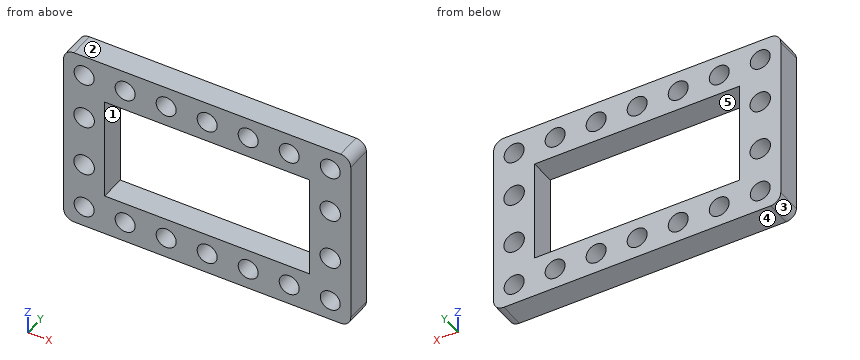
from build123d import *

# Parameters (mm, degrees)
BOSS_EXTRUDE1_DEPTH = 5
SKETCH2_R           = 1.95
SKETCH2_W           = 40
SKETCH2_H           = 20
CUT_EXTRUDE1_DEPTH  = 6
SKETCH4_W           = 22
SKETCH4_H           = 36
CUT_EXTRUDE2_DEPTH  = 10
FILLET1_R           = 2
FILLET2_R           = 2
FILLET3_R           = 2
FILLET4_R           = 2
SKETCH5_R           = 2
CUT_EXTRUDE3_DEPTH  = 6


with BuildPart() as part:
    # Sketch1 → Boss-Extrude1 (new body)
    with BuildSketch(Plane(origin=(0, 0, 0), x_dir=(1, 0, 0), z_dir=(0, 1, 0))):
        with BuildLine():
            Line((2, 0), (98, 0))
            ThreePointArc((98, 0), (99.414213562, -0.585786438), (100, -2))
            Line((100, -2), (100, -34))
            ThreePointArc((100, -34), (99.414213562, -35.414213562), (98, -36))
            Line((98, -36), (2, -36))
            ThreePointArc((2, -36), (0.585786438, -35.414213562), (0, -34))
            Line((0, -34), (0, -2))
            ThreePointArc((0, -2), (0.585786438, -0.585786438), (2, 0))
        make_face()
    extrude(amount=BOSS_EXTRUDE1_DEPTH)

    # Sketch2 → Cut-Extrude1 (cut, through all)
    with BuildSketch(Plane(origin=(0, 5, 0), x_dir=(1, 0, 0), z_dir=(0, 1, 0))):
        with Locations((90, -4.00475022)):
            Circle(SKETCH2_R)
        with Locations((82, -4.00475022)):
            Circle(SKETCH2_R)
        with Locations((18, -4.00475022)):
            Circle(SKETCH2_R)
        with Locations((26, -4.00475022)):
            Circle(SKETCH2_R)
        with Locations((34, -4.00475022)):
            Circle(SKETCH2_R)
        with Locations((42, -4.00475022)):
            Circle(SKETCH2_R)
        with Locations((50, -4.00475022)):
            Circle(SKETCH2_R)
        with Locations((58, -4.00475022)):
            Circle(SKETCH2_R)
        with Locations((66, -4.00475022)):
            Circle(SKETCH2_R)
        with Locations((74, -4.00475022)):
            Circle(SKETCH2_R)
        with Locations((90, -32)):
            Circle(SKETCH2_R)
        with Locations((82, -32)):
            Circle(SKETCH2_R)
        with Locations((18, -32)):
            Circle(SKETCH2_R)
        with Locations((26, -32)):
            Circle(SKETCH2_R)
        with Locations((34, -32)):
            Circle(SKETCH2_R)
        with Locations((42, -32)):
            Circle(SKETCH2_R)
        with Locations((50, -32)):
            Circle(SKETCH2_R)
        with Locations((58, -32)):
            Circle(SKETCH2_R)
        with Locations((66, -32)):
            Circle(SKETCH2_R)
        with Locations((74, -32)):
            Circle(SKETCH2_R)
        with Locations((50, -18)):
            Rectangle(SKETCH2_W, SKETCH2_H)
    extrude(amount=-CUT_EXTRUDE1_DEPTH, mode=Mode.SUBTRACT)

    # Sketch4 → Cut-Extrude2 (cut)
    with BuildSketch(Plane(origin=(0, 5, 0), x_dir=(1, 0, 0), z_dir=(0, 1, 0))):
        with Locations((89, -18)):
            Rectangle(SKETCH4_W, SKETCH4_H)
        with Locations((11, -18)):
            Rectangle(SKETCH4_W, SKETCH4_H)
    extrude(amount=-CUT_EXTRUDE2_DEPTH, mode=Mode.SUBTRACT)

    # Fillet1
    fillet1_edges = [part.edges().sort_by_distance(p)[0] for p in [
        (22, 2.5, 0),
    ]]
    fillet(fillet1_edges, radius=FILLET1_R)

    # Fillet2
    fillet2_edges = [part.edges().sort_by_distance(p)[0] for p in [
        (22, 2.5, 36),
    ]]
    fillet(fillet2_edges, radius=FILLET2_R)

    # Fillet3
    fillet3_edges = [part.edges().sort_by_distance(p)[0] for p in [
        (78, 2.5, 36),
    ]]
    fillet(fillet3_edges, radius=FILLET3_R)

    # Fillet4
    fillet4_edges = [part.edges().sort_by_distance(p)[0] for p in [
        (78, 2.5, 0),
    ]]
    fillet(fillet4_edges, radius=FILLET4_R)

    # Sketch5 → Cut-Extrude3 (cut, through all)
    with BuildSketch(Plane(origin=(0, 5, 0), x_dir=(1, 0, 0), z_dir=(0, 1, 0))):
        with Locations((74, -13)):
            Circle(SKETCH5_R)
        with Locations((74, -23)):
            Circle(SKETCH5_R)
        with Locations((26, -13)):
            Circle(SKETCH5_R)
        with Locations((26, -23)):
            Circle(SKETCH5_R)
    extrude(amount=-CUT_EXTRUDE3_DEPTH, mode=Mode.SUBTRACT)


solid = part.part
Can you work these out from the model? Positions are in its coordinate system, mm. Face numbers are marked on the shaded views. A direction names the side the tool comes from. Round coordinates to 2 decimals unless told otherwise and drop trailing zeros. Order: outer loops, then holes, each group sorted by start corner. A loop starts at its lowest first (then second) coordinate and runs counter-clockwise, first axis right, second up. Notation, with made-up numbers: (-12, -14.75) - (-6, -14.75) arc R20 cw to (-6, 19.25) - close; hole circle Ø2 at (7.25, 52). An arc over 180 degrees is marked (long way). Answer in a Markdown table with one row per item.
(1) Suppose I cut it at D-D, the plane z = 13. Please give me the cut outline in (x, y), plus the area to 3 significant figures.
From the geometry:
| item | result |
|---|---|
| outline | (22, 0) - (24, 0) - (24, 5) - (22, 5) - close; (28, 0) - (30, 0) - (30, 5) - (28, 5) - close; (70, 0) - (72, 0) - (72, 5) - (70, 5) - close; (76, 0) - (78, 0) - (78, 5) - (76, 5) - close |
| area | 40.0 mm2 |
(2) Suppose I cut it at C-C, the plane x = 39. Please give me the cut outline in (y, z).
From the geometry:
| item | result |
|---|---|
| outline | (0, 0) - (5, 0) - (5, 8) - (0, 8) - close; (0, 28) - (5, 28) - (5, 36) - (0, 36) - close |
(3) Please list where these lines run through material, in increasing order: L1, parallel to Z at x = 26, y = 1.45; L2, parallel to Z at x = 50, y = 3; L3, parallel to X at y = 3, z = 27. Write a range as from..to.
From the geometry:
| item | result |
|---|---|
| L1 | z = 0..2.05, 5.95..11, 15..21, 25..30.05, 33.95..36 |
| L2 | z = 0..2.05, 5.95..8, 28..30.05, 33.95..36 |
| L3 | x = 22..30, 70..78 |
(4) Suppose I cut it at A-A, the plane z = 19.5. Please give me the cut outline in (x, y), plus the area to 3 significant figures.
From the geometry:
| item | result |
|---|---|
| outline | (22, 0) - (30, 0) - (30, 5) - (22, 5) - close; (70, 0) - (78, 0) - (78, 5) - (70, 5) - close |
| area | 80.0 mm2 |
(5) Suppose I cut it at B-B, the plane x = 74. Please give me the cut outline in (y, z), plus the area to 3 significant figures.
From the geometry:
| item | result |
|---|---|
| outline | (0, 0) - (5, 0) - (5, 2.05) - (0, 2.05) - close; (0, 5.95) - (5, 5.95) - (5, 11) - (0, 11) - close; (0, 15) - (5, 15) - (5, 21) - (0, 21) - close; (0, 25) - (5, 25) - (5, 30.05) - (0, 30.05) - close; (0, 33.95) - (5, 33.95) - (5, 36) - (0, 36) - close |
| area | 101 mm2 |
(6) Which directions (+Z, -Z, +X, -X, +Y, -Y) give clear straight access to the entire face, cutting with the end or side of a thin tool? Please do the marked faces 1 and 2.
From the geometry:
| item | result |
|---|---|
| face 1 | +Y, -Y |
| face 2 | +Z, +X, -X, +Y, -Y |
(7) If we mould it in two halves opening along X, with no side actions, what happens to the marked faces 3, 4 and 5? For each: released by +X, released by -X, zero draft, split by the parting line, or undercut.
From the geometry:
| item | result |
|---|---|
| face 3 | released by -X |
| face 4 | zero draft |
| face 5 | undercut |
